from build123d import *

# Parameters (mm, degrees)
TORUS_R         = 2
CYLINDER_R      = 20
CYLINDER_DEPTH  = 4
POCKET_DEPTH    = 4.001
FILLET_R        = 3
FILLET001_R     = 3
FILLET002_R     = 3
POCKET001_DEPTH = 5


with BuildPart() as torus:
    # Torus → Torus (revolve)
    with BuildSketch(Plane(origin=(0, 0, 2), x_dir=(1, 0, 0), z_dir=(0, -1, 0))):
        with Locations((20, 0)):
            Circle(TORUS_R)
    revolve(axis=Axis((0, 0, 2), (0, 0, 1)))


with BuildPart() as body001:
    # Cylinder → Cylinder (new body)
    with BuildSketch(Plane.XY):
        Circle(CYLINDER_R)
    extrude(amount=CYLINDER_DEPTH)

    # Sketch001 (on DatumPlane) → Pocket (cut, through all)
    with BuildSketch(Plane(origin=(0, 0, 0), x_dir=(1, 0, 0), z_dir=(0, 0, -1))):
        with BuildLine():
            Line((2, 17), (2, 2))
            Line((2, 2), (17, 2))
            ThreePointArc((17, 2), (12.606602, 12.606602), (2, 17))
        make_face()
        with BuildLine():
            Line((-2, 17), (-2, 2))
            Line((-17, 2), (-2, 2))
            ThreePointArc((-2, 17), (-12.606602, 12.606602), (-17, 2))
        make_face()
        with BuildLine():
            Line((2, -2), (17, -2))
            ThreePointArc((2, -17), (12.606602, -12.606602), (17, -2))
            Line((2, -2), (2, -17))
        make_face()
        with BuildLine():
            Line((-2, -2), (-2, -17))
            ThreePointArc((-17, -2), (-12.606602, -12.606602), (-2, -17))
            Line((-17, -2), (-2, -2))
        make_face()
    extrude(amount=-POCKET_DEPTH, mode=Mode.SUBTRACT)

    # Fillet
    fillet_edges = [body001.edges().sort_by_distance(p)[0] for p in [
        (-2, -17, 2),
    ]]
    fillet(fillet_edges, radius=FILLET_R)

    # Fillet001
    fillet001_edges = [body001.edges().sort_by_distance(p)[0] for p in [
        (-17, 2, 2),
        (2, -17, 2),
        (17, -2, 2),
        (-17, -2, 2),
        (-2, 17, 2),
        (2, 17, 2),
        (17, 2, 2),
    ]]
    fillet(fillet001_edges, radius=FILLET001_R)

    # Fillet002
    fillet002_edges = [body001.edges().sort_by_distance(p)[0] for p in [
        (2, -2, 2),
        (2, 2, 2),
        (-2, 2, 2),
        (-2, -2, 2),
    ]]
    fillet(fillet002_edges, radius=FILLET002_R)

    # Cut: cut Torus
    add(torus.part, mode=Mode.SUBTRACT)

    # Sketch (on DatumPlane) → Pocket001 (cut)
    with BuildSketch(Plane(origin=(0, 0, 0), x_dir=(1, 0, 0), z_dir=(0, 0, -1))):
        Polygon((1.109782, -2.679251), (2.679251, -1.109782), (2.679251, 1.109782), (1.109782, 2.679251), (-1.109782, 2.679251), (-2.679251, 1.109782), (-2.679251, -1.109782), (-1.109782, -2.679251), align=None)
    extrude(amount=-POCKET001_DEPTH, mode=Mode.SUBTRACT)


solid = body001.part
Work out the finished part from the listing and answer in its coordinate system (mm). Give positions to 0.01 mm unless a question says otherwise; leave off trailing zeros. Write each loop counter-clockwise with the first axis right and the second up, starting at its lowest first coordinate (ties: lowest second). Pieces come first, ordered by that corner, then holes.
Q1. Straight lines are drawn through the part: L1, parallel to Y at x = -10, z = 2.3; L2, parallel to Y at x = 12.5, z = 2.7; L3, parallel to X at y = 7.5, z = 0.35. For each, find the intervals that lie inside material, in ascending order.
Answer:
L1: y = -14.99 to -14.69, -2 to 2, 14.69 to 14.99
L2: y = -13.13 to -12.71, -2 to 2, 12.71 to 13.13
L3: x = -17.32 to -15.96, -2 to 2, 15.96 to 17.32
Q2. For a pull along Y with two mould halves and no side action, classify faces 1 (the face through (0, -4, 0)), 2 (the face through (9, 2, 2)) as released by +Y, released by -Y, zero draft, split by the parting line, or undercut.
Answer:
face 1: zero draft
face 2: undercut
Q3. The part is cut by section A-A on x = 0. Give the vertices of the cut face in (y, z), and give its area (3 significant figures).
Answer:
outline: (-20, 0) - (-2.68, 0) - (-2.68, 4) - (-20, 4) arc R2 cw to start; (2.68, 0) - (20, 0) arc R2 cw to (20, 4) - (2.68, 4) - close
area: 126 mm2
Q4. Given pin 1 (1.1 mm diameter, centred on y = 0, z = 2.5, fed in from +X); pin 2 (1.2 mm diameter, centred on x = 7.5, z = 1, fed in from +Y); pin 3 (2 mm diameter, centred on y = -10.5, z = 1.5, fed in from -X), each flat-ended and moving along its own axis, determine where each tip first touches the part or whether it passes through.
Answer:
pin 1: stops at x = 18.3
pin 2: stops at y = 17.28
pin 3: stops at x = -15.61
Q5. The part is cut by section B-B on z = 2.1. State how many separate pieces and enclosed holes the cut face has, and give its area (3 significant figures).
Answer:
separate pieces: 1
enclosed holes: 5
area: 318 mm2
